```python
from build123d import *

# Parameters (mm, degrees)
SKETCH1_R                 = 5
SKETCH1_R_2               = 3
BOSS_EXTRUDE1_DEPTH       = 14
BOSS_EXTRUDE2_DEPTH       = 4
M3_CLEARANCE_HOLE1_D      = 3.4
M3_CLEARANCE_HOLE2_REACH  = 25.495
M3_CLEARANCE_HOLE2_BORE_R = 1.7
BOSS_EXTRUDE3_REACH       = 25.495
BOSS_EXTRUDE3_END_RADIUS  = 5
SKETCH11_R                = 2.549362178
SKETCH11_R_2              = 1.7
SKETCH14_R                = 2.549362178
CUT_EXTRUDE2_DEPTH        = 1
BOSS_EXTRUDE4_DEPTH       = 2


with BuildPart() as part:
    # Sketch1 → Boss-Extrude1 (new body)
    with BuildSketch(Plane(origin=(0, 0, 0), x_dir=(1, 0, 0), z_dir=(0, 1, 0))):
        with Locations(Location((0, 0, 0), (0, 0, 270))):
            Circle(SKETCH1_R)
        with Locations(Location((0, 0, 0), (0, 0, 270))):
            Circle(SKETCH1_R_2, mode=Mode.SUBTRACT)
    extrude(amount=BOSS_EXTRUDE1_DEPTH)

    # Sketch2 → Boss-Extrude2 (add)
    with BuildSketch(Plane(origin=(0, 14, 0), x_dir=(1, 0, 0), z_dir=(0, 1, 0))):
        Polygon((0, 6.92820323), (-6, 3.464101615), (-6, -3.464101615), (0, -6.92820323), (6, -3.464101615), (6, 3.464101615), align=None)
    extrude(amount=BOSS_EXTRUDE2_DEPTH)

    # M3 Clearance Hole1 (through all)
    with Locations(Plane(origin=(0, 18, 0), x_dir=(1, 0, 0), z_dir=(0, 1, 0))):
        with Locations((0, 0)):
            Hole(M3_CLEARANCE_HOLE1_D / 2)

    # M3 Clearance Hole2 bore → M3 Clearance Hole2 (cut, up to next)
    with BuildSketch(Plane(origin=(-3, 0, -5.196152423), x_dir=(-0.8660254037844386, 0, 0.5000000000000003), z_dir=(-0.5000000000000002, 0, -0.8660254037844385)), mode=Mode.PRIVATE) as m3_clearance_hole2_sk1:
        with Locations((0, 6)):
            Circle(M3_CLEARANCE_HOLE2_BORE_R)
    m3_clearance_hole2_tool1 = extrude(m3_clearance_hole2_sk1.sketch, amount=-M3_CLEARANCE_HOLE2_REACH, mode=Mode.PRIVATE) & part.part
    add(m3_clearance_hole2_tool1.solids().sort_by_distance((-3, 6, -5.196152))[0], mode=Mode.SUBTRACT)

    # Boss-Extrude3: up to this cylinder (the profile starts outside it)
    boss_extrude3_end = Plane(origin=(0, 6, 0), z_dir=(0, -1, 0)) * Cylinder(BOSS_EXTRUDE3_END_RADIUS, 61.99, mode=Mode.PRIVATE)
    # Sketch11 → Boss-Extrude3 (add, up to the surface)
    with BuildSketch(Plane(origin=(-3, 0, -5.196152423), x_dir=(-0.8660254037844386, 0, 0.5000000000000003), z_dir=(-0.5000000000000002, 0, -0.8660254037844385)), mode=Mode.PRIVATE) as boss_extrude3_sk1:
        with Locations((0, 6)):
            Circle(SKETCH11_R)
        with Locations((0, 6)):
            Circle(SKETCH11_R_2, mode=Mode.SUBTRACT)
    boss_extrude3_tool1 = extrude(boss_extrude3_sk1.sketch, amount=-BOSS_EXTRUDE3_REACH, mode=Mode.PRIVATE) - boss_extrude3_end
    add(boss_extrude3_tool1.solids().sort_by_distance((-0.854634, 6, -6.43478))[0])

    # Sketch14 → Cut-Extrude2 (cut)
    with BuildSketch(Plane(origin=(-3, 0, -5.196152423), x_dir=(-0.8660254037844384, 0, 0.5000000000000004), z_dir=(-0.5000000000000004, 0, -0.8660254037844384))):
        with Locations((0, 6)):
            Circle(SKETCH14_R)
    extrude(amount=-CUT_EXTRUDE2_DEPTH, mode=Mode.SUBTRACT)

    # Sketch19 → Boss-Extrude4 (add)
    with BuildSketch(Plane.XZ.offset(-14)):
        Polygon((0, -6.92820323), (6, -3.464101615), (6, 3.464101615), (0, 6.92820323), (-6, 3.464101615), (-6, -3.464101615), align=None)
    extrude(amount=BOSS_EXTRUDE4_DEPTH)


solid = part.part
```
Verification items for the finished model (mm, model axes). A direction names the side the tool comes from. Give positions to 0.01 mm unless a question says otherwise; leave off trailing zeros. Loops run counter-clockwise (first coordinate to the right, second up) from the corner with the lowest first, then second, coordinate; pieces in that order, holes last.
1. Mould release check, pull along Z, two halves, no side actions. Record for faces 5 (the flat face through (2.96, 15.04, -5.22)), 6 (the flat face through (-6, 15, 0)), 7 (the flat face through (3.042, 15.042, 5.172)), 8 (the cylindrical face through (-4.57, 5.94, -2.82)): released by +Z, released by -Z, zero draft, split by the parting line, or undercut.
2. Set-up check for faces 1 (the cylindrical face through (-0.159, 6.056, -5.373)), 2 (the flat face through (-3.3, 0, -0.1)), 3 (the flat face through (0, 14, 0)), 4 (the flat face through (0, 12, 0)): record each of +Z, -Z, +X, -X, +Y, -Y from which the full face is reachable in a straight line by a thin tool's end or side.
3. Go/stop test with flat-tipped pins: pin 1 Ø3 at (y, z) = (6.5, -4.5) entering from -X; pin 2 Ø2.5 at (x, z) = (0, 0) entering from +Y; pin 3 Ø1.5 at (y, z) = (9.5, -3) entering from +X. Record where each tip stops, or that it passes through.
4. Section check A-A, the plane y = 2. Enter the section's corners in (x, z), then the cut area to 3 significant figures.
5. Section check C-C, the plane x = 4.75. Enter the section's corners in (y, z).
6. Section check B-B, the plane y = 7. Enter the section's corners in (x, z).
7. Thickness scan on line 1 (Z direction, x = 0, y = 5); line 2 (Z direction, x = 0, y = 5.25). Record the ranges inside material, lowest first.
Geometry says:
1. face 5: released by -Z
1. face 6: zero draft
1. face 7: released by +Z
1. face 8: undercut
2. face 1: -Z
2. face 2: +Z, -Z, +X, -X, -Y
2. face 3: +Y
2. face 4: -Y
3. pin 1: stops at x = -4.71
3. pin 2: stops at y = 14
3. pin 3: stops at x = 4.47
4. outline: circle Ø10 at (0, 0); hole circle Ø6 at (0, 0)
4. area: 50.3 mm2
5. outline: (0, -1.56) - (12, -1.56) - (12, -4.19) - (18, -4.19) - (18, 4.19) - (12, 4.19) - (12, 1.56) - (0, 1.56) - close
6. outline: (-4.53, -3.16) - (-3.69, -3.64) - (-2.52, -1.62) arc R3 cw (long way) to (-0.14, -3) - (-1.31, -5.02) - (-0.47, -5.5) - (-0.18, -5) arc R5 ccw (long way) to (-4.24, -2.65) - close
7. line 1: z = -5 to -3, 3 to 5
7. line 2: z = -5 to -3.05, 3 to 5
